from build123d import *

# Parameters (mm, degrees)
SKETCH1_W                 = 96.210678118
SKETCH1_H                 = 96.210678118
SKETCH1_R                 = 4.25
SKETCH1_R_2               = 9
BODY_AND_MAIN_HOLES_DEPTH = 14
SKETCH2_R                 = 10
SEAL_HOLE_DEPTH           = 6
BEARING_START             = -6
SKETCH3_R                 = 10
BEARING_HOLE_DEPTH        = 6
SKETCH4_R                 = 2
CUT_EXTRUDE1_DEPTH        = 10


with BuildPart() as part:
    # Sketch1 → body and main holes (new body)
    with BuildSketch(Plane(origin=(0, 0, 0), x_dir=(1, 0, 0), z_dir=(0, 1, 0))):
        Rectangle(SKETCH1_W, SKETCH1_H)
        with Locations(Location((-35.355339059, 35.355339059, 0), (0, 0, 270))):
            Circle(SKETCH1_R, mode=Mode.SUBTRACT)
        with Locations(Location((35.355339059, 35.355339059, 0), (0, 0, 270))):
            Circle(SKETCH1_R, mode=Mode.SUBTRACT)
        with Locations(Location((35.355339059, -35.355339059, 0), (0, 0, 270))):
            Circle(SKETCH1_R, mode=Mode.SUBTRACT)
        with Locations(Location((-35.355339059, -35.355339059, 0), (0, 0, 270))):
            Circle(SKETCH1_R, mode=Mode.SUBTRACT)
        with Locations(Location((0, 0, 0), (0, 0, 270))):
            Circle(SKETCH1_R_2, mode=Mode.SUBTRACT)
    extrude(amount=BODY_AND_MAIN_HOLES_DEPTH)

    # Sketch2 → seal hole (cut)
    with BuildSketch(Plane(origin=(0, 14, 0), x_dir=(1, 0, 0), z_dir=(0, 1, 0))):
        with Locations(Location((0, 0, 0), (0, 0, 270))):
            Circle(SKETCH2_R)
    extrude(amount=-SEAL_HOLE_DEPTH, mode=Mode.SUBTRACT)

    # Sketch3 → bearing hole (cut)
    with BuildSketch(Plane.XZ.offset(BEARING_START)):
        with Locations(Location((0, 0, 0), (0, 0, 90))):
            Circle(SKETCH3_R)
    extrude(amount=BEARING_HOLE_DEPTH, mode=Mode.SUBTRACT)

    # Sketch4 → Cut-Extrude1 (cut)
    with BuildSketch(Plane.XZ):
        with Locations(Location((0, -15, 0), (0, 0, 270))):
            Circle(SKETCH4_R)
        with Locations(Location((-15, 0, 0), (0, 0, 270))):
            Circle(SKETCH4_R)
        with Locations(Location((0, 15, 0), (0, 0, 270))):
            Circle(SKETCH4_R)
        with Locations(Location((15, 0, 0), (0, 0, 270))):
            Circle(SKETCH4_R)
    extrude(amount=-CUT_EXTRUDE1_DEPTH, mode=Mode.SUBTRACT)


solid = part.part
Design review of the part built by this model. Coordinates are the model's own, in mm. A direction names the side the tool comes from. Coordinates: 2 decimals unless noted, no trailing zeros. Write each loop counter-clockwise with the first axis right and the second up, starting at its lowest first coordinate (ties: lowest second). Pieces come first, ordered by that corner, then holes. Notation, with made-up numbers: (18.25, 42) -> (70.25, 42) arc R13 ccw to (70.25, 57) -> close; hole circle Ø9 at (-35.75, 53). An arc over 180 degrees is marked (long way). Write each question's results on one line, items separated by ' | '. Start each with the question number.
(1) Take a section at D-D on y = 12. Write out the cut boundary in (x, z), and give its area (3 significant figures).
(2) Take a section at C-C on x = 15. Write out the cut boundary in (y, z), and give its area (3 significant figures).
(3) For line 1 along X through (y, z) = (7.25, 0); line 2 along X through (y, z) = (10.8, 0); line 3 along X through (y, z) = (4, 0), list the stretches that pass through material, from the lowest coordinate up. Write a range as from..to.
(4) Take a section at A-A on x = 0. Write out the cut boundary in (y, z).
(5) Tool access review of faces 4 (the face through (-9.76, 11.04, -2.17)), 5 (the face through (-15, 10, 0)), 6 (the face through (-1, 7, 48.105)): name each direction out of +Z, -Z, +X, -X, +Y, -Y from which nothing blocks a thin tool from reaching the whole face with its end or side.
(6) Take a section at B-B on z = 0. Write out the cut boundary in (x, y).
(7) The part is to be moulded in two halves that separate along Z. For faces 1 (the face through (-13, 5, 0)), 2 (the face through (-1, 7, -48.105)), 3 (the face through (-1, 14, -11)), say which applies: pulls with the +Z half, pulls with the -Z half, needs draft (parallel to the pull), parting line crosses it, or undercut.
(8) Clearance check with flat-ended pins moving along their axes: P1, Ø3, axis at x = 0.5, z = -14.5, coming from the -Y side; P2, Ø2.5, axis at x = -15, z = 0, coming from the -Y side; P3, Ø5, axis at x = -35.36, z = 35.36, coming from the +Y side. State where each tip first meets the part, or that it passes through.
Results found:
1) outline: (-48.11, -48.11) -> (48.11, -48.11) -> (48.11, 48.11) -> (-48.11, 48.11) -> close; hole circle Ø8.5 at (-35.36, -35.36); hole circle Ø8.5 at (-35.36, 35.36); hole circle Ø20 at (0, 0); hole circle Ø8.5 at (35.36, -35.36); hole circle Ø8.5 at (35.36, 35.36) | area: 8,720 mm2
2) outline: (0, -48.11) -> (14, -48.11) -> (14, 48.11) -> (0, 48.11) -> (0, 2) -> (10, 2) -> (10, -2) -> (0, -2) -> close | area: 1,310 mm2
3) line 1: x = -48.11..-17, -13..-9, 9..13, 17..48.11 | line 2: x = -48.11..-10, 10..48.11 | line 3: x = -48.11..-17, -13..-10, 10..13, 17..48.11
4) outline: (0, -48.11) -> (14, -48.11) -> (14, -10) -> (8, -10) -> (8, -9) -> (6, -9) -> (6, -10) -> (0, -10) -> (0, -13) -> (10, -13) -> (10, -17) -> (0, -17) -> close; (0, 10) -> (6, 10) -> (6, 9) -> (8, 9) -> (8, 10) -> (14, 10) -> (14, 48.11) -> (0, 48.11) -> (0, 17) -> (10, 17) -> (10, 13) -> (0, 13) -> close
5) face 4: +Y | face 5: -Y | face 6: +Z, +X, -X, +Y, -Y
6) outline: (-48.11, 0) -> (-17, 0) -> (-17, 10) -> (-13, 10) -> (-13, 0) -> (-10, 0) -> (-10, 6) -> (-9, 6) -> (-9, 8) -> (-10, 8) -> (-10, 14) -> (-48.11, 14) -> close; (9, 6) -> (10, 6) -> (10, 0) -> (13, 0) -> (13, 10) -> (17, 10) -> (17, 0) -> (48.11, 0) -> (48.11, 14) -> (10, 14) -> (10, 8) -> (9, 8) -> close
7) face 1: undercut | face 2: pulls with the -Z half | face 3: needs draft
8) P1: stops at y = 0 | P2: stops at y = 10 | P3: passes through
